Geometry: final body of the model. Coordinates: model frame, mm. A direction names the side the tool comes from. Round coordinates to 2 decimals unless told otherwise and drop trailing zeros. Order: outer loops, then holes, each group sorted by start corner. A loop starts at its lowest first (then second) coordinate and runs counter-clockwise, first axis right, second up. Notation, with made-up numbers: (-25, 22) - (-11, 22) arc R28 ccw to (-11, 52) - close; hole circle Ø2 at (58.5, -6). An arc over 180 degrees is marked (long way). Put each result on its own line as item: value. Start each with the question number.
(1) Section A-A (y = 24). Output: boundary loops of the cut face in (x, z) (3 decimals).
(2) Pin query (flat end, axial travel): P1, Ø2, axis at y = 40, z = 20, coming from the -X side; P2, Ø12, axis at y = 31.5, z = 10, coming from the +X side; P3, Ø4, axis at y = 7.5, z = -13.5, coming from the +X side; P4, Ø6, axis at x = 0.5, y = 22, coming from the +Z side. Return the tip coordinate at first contact, or that it passes through.
(3) Access query for faces 1 (the face through (18.74, 38.32, 11.95)), 2 (the face through (-53.975, 17, 13)), 3 (the face through (-22.225, 5, -17)). Directions: +Z, -Z, +X, -X, +Y, -Y. A direction counts if a zero-diameter tool reaches every point of the face in a straight line with its end or side. Return the directions, or none.
(4) Material intervals for L1, parallel to X at y = 43.5, z = 0 (3 decimals); L2, parallel to Y at x = -36, z = -4; L3, parallel to Z at x = -39.5, y = 12, sorted ascending. Write a range as [from, to].
(5) Section B-B (y = 42). Output: boundary loops of the cut face in (x, z) (3 decimals).
(6) Pull-direction query (Z, two-part tool) for faces 4 (the face through (17, 53.975, -15)), 5 (the face through (-37.88, -21.2, 13.52)), 6 (the face through (-38.32, -6.34, 20.14)); classes: released by +Z, released by -Z, zero draft, split by the parting line, or undercut.
from build123d import *

# Parameters (mm, degrees)
SKETCH3_R          = 25.146
SKETCH3_R_2        = 17.526
SKETCH5_R          = 22.225
CUT_EXTRUDE1_DEPTH = 31.75


with BuildPart() as part:
    # Sketch1 → Revolve1 (revolve)
    with BuildSketch(Plane.XY, mode=Mode.PRIVATE) as revolve1_sk:
        Polygon((-53.975, -25.146), (-22.225, -25.146), (-22.225, -21.0185), (-53.975, -21.209), align=None)
    revolve(revolve1_sk.sketch.rotate(Axis((-53.975, 0, 0), (1, 0, 0)), 270), axis=Axis((-53.975, 0, 0), (1, 0, 0)))


with BuildPart() as body_2:
    # Sketch2 → Revolve2 (revolve)
    with BuildSketch(Plane.XY, mode=Mode.PRIVATE) as revolve2_sk:
        Polygon((21.209, 53.975), (21.0185, 22.225), (25.146, 22.225), (25.146, 53.975), align=None)
    revolve(revolve2_sk.sketch.rotate(Axis((0, 0, 0), (0, 1, 0)), 90), axis=Axis((0, 0, 0), (0, 1, 0)))


with BuildPart() as sweep1_tool:
    # Sweep1: sweep along a path in Sketch4
    with BuildLine(Plane.XY) as sweep1_path:
        ThreePointArc((-22.225, 0), (-6.509552, 6.509552), (0, 22.225))
    # Sketch3 → Sweep1 (sweep)
    with BuildSketch(Plane(origin=(-22.225, 0, 0), x_dir=(0, 0, -1), z_dir=(1, 0, 0))):
        Circle(SKETCH3_R)
        Circle(SKETCH3_R_2, mode=Mode.SUBTRACT)
    sweep(path=sweep1_path.line)


with BuildPart() as part_1:
    add(part.part)


with BuildPart() as part_2:
    # Sweep1: joined with sweep1_tool
    add(part_1.part.fuse(sweep1_tool.part, body_2.part, tol=0.00001))

    # Sketch5 → Cut-Extrude1 (cut)
    with BuildSketch(Plane(origin=(0, 53.975, 0), x_dir=(1, 0, 0), z_dir=(0, 1, 0))):
        with Locations(Location((0, 0, 0), (0, 0, 270))):
            Circle(SKETCH5_R)
    extrude(amount=-CUT_EXTRUDE1_DEPTH, mode=Mode.SUBTRACT)


solid = part_2.part
Checks:
1. outline: (-53.975, -7.505) - (-24, -7.505) arc R25.146 ccw (long way) to (-24, 7.505) - (-53.975, 7.505) - close; hole circle Ø44.45 at (0, 0)
2. P1: stops at x = -16.47
2. P2: stops at x = 24.83
2. P3: stops at x = 20.05
2. P4: stops at z = 25.15
3. face 1: +Y
3. face 2: +Z, -Z, -X, +Y, -Y
3. face 3: -X
4. L1: x = [-25.146, -22.225], [22.225, 25.146]
4. L2: y = [-24.83, -20.72], [20.72, 24.83]
4. L3: z = [-22.1, -17.38], [17.38, 22.1]
5. outline: circle Ø50.292 at (0, 0); hole circle Ø44.45 at (0, 0)
6. face 4: zero draft
6. face 5: split by the parting line
6. face 6: undercut
